Input: part model. Units: mm. Frame: model coordinates. A direction names the side the tool comes from. Round coordinates to 2 decimals unless told otherwise and drop trailing zeros. Loops run counter-clockwise (first coordinate to the right, second up) from the corner with the lowest first, then second, coordinate; pieces in that order, holes last. Notation, with made-up numbers: (61, 68.5) -> (87, 68.5) arc R15 ccw to (87, 95.5) -> close; hole circle Ø3 at (67.25, -33). An arc over 180 degrees is marked (long way). Answer in a Markdown table with one row per item. Add a question column.
Q1. Pin query (flat end, axial travel): pin 1 (3 mm diameter, centred on x = 78, z = 4, fed in from +Y); pin 2 (8 mm diameter, centred on x = 57.5, y = 0.5, fed in from +Z); pin 3 (7.5 mm diameter, centred on x = -26, y = 2.5, fed in from +Z). Return the tip coordinate at first contact, or that it passes through.
Q2. Section D-D, the plane x = -15. Output: boundary loops of the cut face in (y, z), and give its area (3 significant figures).
Q3. Section B-B, the plane x = 136. Output: boundary loops of the cut face in (y, z).
Q4. Ray query, L1, parallel to X at y = 0.75, z = -2.75; L2, parallel to Y at x = 22, z = 2.25; L3, parallel to X at y = 0.5, z = 2.5. Return the intervals inside material, ascending. Write a range as from..to.
Q5. Section A-A, the plane z = 0. Output: boundary loops of the cut face in (x, y).
Q6. Reachability of faces 1 (the face through (-20, 0, -2.65)), 2 (the face through (144.101, 5.158, 3.955)), 3 (the face through (-20, 0, 2.65)), 4 (the face through (-5.777, -3.428, -1.079)), 5 (the face through (53.812, 2.583, 4.534)) from +Z, -Z, +X, -X, +Y, -Y: full face, straight path, thin tool, end or side. Return the list, or none.
Q7. Section C-C, the plane x = 69. Output: boundary loops of the cut face in (y, z).
Q8. Mould query, pull axis X, two halves, no side actions, for faces 6 (the face through (137.497, -1.54, -4.42)), 7 (the face through (-29.213, -2.805, 0.037)), 8 (the face through (53.812, 2.635, -4.503)). Classes: pulls with the +X half, pulls with the -X half, needs draft (parallel to the pull), parting line crosses it, or undercut.
```python
from build123d import *

# Parameters (mm, degrees)
F0_W     = 1.7
F0_H     = 2
F0_W_2   = 26
F0_H_2   = 5
F0_W_3   = 54
F0_H_3   = 6
F0_W_4   = 47
F0_H_4   = 4.5
F2_DEPTH = 2.65
F4_DEPTH = 97.7


with BuildPart() as f1:
    # F0 (on Top) → F1 (revolve)
    with BuildSketch(Plane.XY):
        with Locations((-6.814198, -1)):
            Rectangle(F0_W, F0_H)
        with Locations((10.035802, -2.5)):
            Rectangle(F0_W_2, F0_H_2)
        Polygon((25.035802, 0), (23.035802, 0), (23.035802, -5), (25.035802, -6), align=None)
        with Locations((52.035802, -3)):
            Rectangle(F0_W_3, F0_H_3)
        Polygon((90.496607, 0), (79.035802, 0), (79.035802, -6), (90.496607, -4.5), align=None)
        with Locations((113.996607, -2.25)):
            Rectangle(F0_W_4, F0_H_4)
        Polygon((150.523409, 0), (137.496607, 0), (137.496607, -4.5), (137.496607, -6.5), (150.523409, -6.5), align=None)
        Polygon((-2.964198, 0), (-5.964198, 0), (-5.964198, -2), (-5.964198, -3.5), (-2.964198, -5), align=None)
    revolve(axis=Axis((44.526573, 0, 0), (1, 0, 0)))

    # F0 (on Top) → F2 (join, symmetric)
    with BuildSketch(Plane.XY):
        Polygon((-7.664198, 7.5), (-29.664198, 7.5), (-32.664198, 1.760973), (-25.664198, -7.5), (-7.664198, -7.5), (-7.664198, -2), (-7.664198, 0), align=None)
    extrude(amount=F2_DEPTH, both=True)

    # F3 (on Right) → F4 (cut)
    with BuildSketch(Plane.YZ):
        Polygon((0.013024, 7.701685), (0.013024, 6.024447), (5.223836, 3.000944), (8.659112, 3.000944), (8.659112, -3.023503), (5.210811, -3.023503), (-0.013024, -6.024447), (0.013024, -7.905965), (11.633459, -7.905965), (11.633459, 7.701685), align=None)
    extrude(amount=F4_DEPTH, mode=Mode.SUBTRACT)


solid = f1.part
```
Answer block:
| question | item | result |
|---|---|---|
| 1 | pin 1 | y = 5.45 |
| 1 | pin 2 | z = 6 |
| 1 | pin 3 | z = 2.65 |
| 2 | outline | (-7.5, -2.65) -> (7.5, -2.65) -> (7.5, 2.65) -> (-7.5, 2.65) -> close |
| 2 | area | 79.5 mm^2 |
| 3 | outline | circle Ø9 at (0, 0) |
| 4 | L1 | -5.96..150.52 |
| 4 | L2 | -4.47..4.47 |
| 4 | L3 | -31.71..-7.66, -5.96..150.52 |
| 5 | outline | (-32.66, 1.76) -> (-25.66, -7.5) -> (-7.66, -7.5) -> (-7.66, -2) -> (-5.96, -2) -> (-5.96, -3.5) -> (-2.96, -5) -> (23.04, -5) -> (25.04, -6) -> (79.04, -6) -> (90.5, -4.5) -> (137.5, -4.5) -> (137.5, -6.5) -> (150.52, -6.5) -> (150.52, 6.5) -> (137.5, 6.5) -> (137.5, 4.5) -> (90.5, 4.5) -> (79.04, 6) -> (25.04, 6) -> (23.04, 5) -> (-2.96, 5) -> (-5.96, 3.5) -> (-5.96, 2) -> (-7.66, 2) -> (-7.66, 7.5) -> (-29.66, 7.5) -> close |
| 6 | face 1 | -Z, -X, +Y, -Y |
| 6 | face 2 | +X |
| 6 | face 3 | +Z, -X, +Y, -Y |
| 6 | face 4 | none |
| 6 | face 5 | +Z, -X, +Y |
| 7 | outline | (0.03, -6) -> (5.17, -3.05) arc R6 ccw to (5.18, 3.03) -> (0.06, 6) arc R6 ccw (long way) to start |
| 8 | face 6 | undercut |
| 8 | face 7 | pulls with the -X half |
| 8 | face 8 | needs draft |
